Autodesk Inventor part; units mm, degrees
ref_plane "YZ Plane" through (0, 0, 0) normal (1, 0, 0) x (0, 1, 0)
ref_plane "XZ Plane" through (0, 0, 0) normal (0, 1, 0) x (-1, 0, 0)
ref_plane "XY Plane" through (0, 0, 0) normal (0, 0, 1) x (1, 0, 0)
sketch "Sketch1" plane through (0, 0, 0) normal (0, 0, 1) x (1, 0, 0)
  line L0 (-13.35, 6.2) -> (13.35, 6.2)
  line L1 (15.35, 4.2) -> (15.35, -4.2)
  line L2 (13.35, -6.2) -> (-13.35, -6.2)
  line L3 (-15.35, -4.2) -> (-15.35, 4.2)
  line L4 (-15.35, 6.2) -> (15.35, -6.2) construction
  line L5 (15.35, 6.2) -> (-15.35, -6.2) construction
  arc A0 (-13.35, 6.2) -> (-15.35, 4.2) centre (-13.35, 4.2) ccw
  arc A1 (15.35, 4.2) -> (13.35, 6.2) centre (13.35, 4.2) ccw
  arc A2 (13.35, -6.2) -> (15.35, -4.2) centre (13.35, -4.2) ccw
  arc A3 (-15.35, -4.2) -> (-13.35, -6.2) centre (-13.35, -4.2) ccw
  point P0 (0, 0)
  dimension "d0" = 12.4
  dimension "d1" = 30.7
  dimension "d2" = 2
extrude "Extrusion1" add sketch "Sketch1" along normal blind 1
sketch "Sketch2" plane through (0, 0, 1) normal (0, 0, 1) x (1, 0, 0)
  circle A0 centre (-12.495, 0) radius 1.55
  circle A1 centre (12.495, 0) radius 1.55
  line L0 (0, 0) -> (0, 2.0374)
  dimension "d5" = 3.1
  dimension "d6" = 24.99
extrude "Extrusion2" cut sketch "Sketch2" against normal through all
sketch "Sketch3" plane through (0, 0, 1) normal (0, 0, 1) x (1, 0, 0)
  line L0 (6.2132, 4.2657) -> (-6.2132, 4.2657)
  line L1 (-8.2003, 2.0385) -> (-7.7028, -2.3115)
  line L2 (-5.7157, -4.0843) -> (5.7157, -4.0843)
  line L3 (7.7028, -2.3115) -> (8.2003, 2.0385)
  line L4 (0, 0) -> (0, 9.8528)
  arc A0 (-6.2132, 4.2657) -> (-8.2003, 2.0385) centre (-6.2132, 2.2657) ccw
  arc A1 (8.2003, 2.0385) -> (6.2132, 4.2657) centre (6.2132, 2.2657) ccw
  arc A2 (5.7157, -4.0843) -> (7.7028, -2.3115) centre (5.7157, -2.0843) ccw
  arc A3 (-7.7028, -2.3115) -> (-5.7157, -4.0843) centre (-5.7157, -2.0843) ccw
  line L5 (6.2132, 2.2657) -> (-5.7157, -2.0843)
  line L6 (-6.2132, 2.2657) -> (5.7157, -2.0843)
  line L7 (-6.2132, 3.2657) -> (6.2132, 3.2657)
  arc A4 (7.2067, 2.1521) -> (6.2132, 3.2657) centre (6.2132, 2.2657) ccw
  line L8 (7.2067, 2.1521) -> (6.7092, -2.1979)
  arc A5 (5.7157, -3.0843) -> (6.7092, -2.1979) centre (5.7157, -2.0843) ccw
  line L9 (5.7157, -3.0843) -> (-5.7157, -3.0843)
  arc A6 (-6.7092, -2.1979) -> (-5.7157, -3.0843) centre (-5.7157, -2.0843) ccw
  line L10 (-6.7092, -2.1979) -> (-7.2067, 2.1521)
  arc A7 (-6.2132, 3.2657) -> (-7.2067, 2.1521) centre (-6.2132, 2.2657) ccw
  point P0 (8.455, 4.2657)
  point P1 (-8.455, 4.2657)
  point P2 (-7.5, -4.0843)
  point P3 (7.5, -4.0843)
  dimension "d9" = 8.35
  dimension "d10" = 16.91
  dimension "d11" = 15
  dimension "d12" = 2
  dimension "d15" = 1
extrude "Extrusion3" add sketch "Sketch3" along normal blind 6.1
properties part number "Dsub_9pin_female" material "Aluminum 6061"
Read the model definition and answer for the solid it produces. Units are mm, in the model's axes. A direction names the side the tool comes from. Coordinates: 2 decimals unless noted, no trailing zeros. Write each loop counter-clockwise with the first axis right and the second up, starting at its lowest first coordinate (ties: lowest second). Pieces come first, ordered by that corner, then holes. Notation, with made-up numbers: (42.25, 53.5) -> (82.25, 53.5) arc R32 cw to (82.25, 82.5) -> close; hole circle Ø8 at (33.5, 6.5). An arc over 180 degrees is marked (long way). Answer as a JSON object with one key per item and string values.
Q1. The part is cut by section D-D on x = -4. Give the vertices of the cut face in (y, z).
The answers:
{"outline": "(-6.2, 0) -> (6.2, 0) -> (6.2, 1) -> (4.27, 1) -> (4.27, 7.1) -> (3.27, 7.1) -> (3.27, 1) -> (-3.08, 1) -> (-3.08, 7.1) -> (-4.08, 7.1) -> (-4.08, 1) -> (-6.2, 1) -> close"}
Q2. The part is cut by section A-A on y = 1. Give the vertices of the cut face in (x, z).
The answers:
{"outline": "(-15.35, 0) -> (-13.68, 0) -> (-13.68, 1) -> (-15.35, 1) -> close; (-11.31, 0) -> (11.31, 0) -> (11.31, 1) -> (8.08, 1) -> (8.08, 7.1) -> (7.07, 7.1) -> (7.07, 1) -> (-7.07, 1) -> (-7.07, 7.1) -> (-8.08, 7.1) -> (-8.08, 1) -> (-11.31, 1) -> close; (13.68, 0) -> (15.35, 0) -> (15.35, 1) -> (13.68, 1) -> close"}
Q3. A tool of negligible diameter and unlimited length cuts with its end or side. For faces 4 (the cylindrical face through (-7.03, -3.59, 4.01)), 5 (the flat face through (0, 0, 1)), 6 (the cylindrical face through (-14.78, 5.6, 0.49)), from which of +Z, -Z, +X, -X, +Y, -Y can it reach the whole face along a straight path? Write none if from no direction.
The answers:
{"face 4": "+Z, -X, -Y", "face 5": "+Z", "face 6": "+Z, -Z, -X, +Y"}
Q4. The part is cut by section B-B on x = 11.5. Give the vertices of the cut face in (y, z), then the cut area to 3 significant figures.
The answers:
{"outline": "(-6.2, 0) -> (-1.19, 0) -> (-1.19, 1) -> (-6.2, 1) -> close; (1.19, 0) -> (6.2, 0) -> (6.2, 1) -> (1.19, 1) -> close", "area": "10.0 mm2"}
Q5. Consider line 1 (Y direction, x = 2, z = 6.25); line 2 (Z direction, x = 4, y = -4.25); line 3 (X direction, y = 1, z = 3). Determine where each line is inside the solid, lowest interval first. Write a range as [from, to].
The answers:
{"line 1": "y = [-4.08, -3.08], [3.27, 4.27]", "line 2": "z = [0, 1]", "line 3": "x = [-8.08, -7.07], [7.07, 8.08]"}
Q6. The part is cut by section C-C on z = 3.75. Give the vertices of the cut face in (x, y), then the cut area to 3 significant figures.
The answers:
{"outline": "(-8.2, 2.04) -> (-7.7, -2.31) arc R2 ccw to (-5.72, -4.08) -> (5.72, -4.08) arc R2 ccw to (7.7, -2.31) -> (8.2, 2.04) arc R2 ccw to (6.21, 4.27) -> (-6.21, 4.27) arc R2 ccw to start; hole (-7.21, 2.15) -> (-6.71, -2.2) arc R1 ccw to (-5.72, -3.08) -> (5.72, -3.08) arc R1 ccw to (6.71, -2.2) -> (7.21, 2.15) arc R1 ccw to (6.21, 3.27) -> (-6.21, 3.27) arc R1 ccw to start", "area": "42.0 mm2"}
Q7. Flat-ended cylindrical pins translate along their axes: pin 1 Ø2 at (x, z) = (1, 5.5) entering from +Y; pin 2 Ø1.8 at (x, z) = (1.5, 5) entering from -Y. Find the tip coordinate at first contact, or state that the pin passes through.
The answers:
{"pin 1": "stops at y = 4.27", "pin 2": "stops at y = -4.08"}
Q8. Determine the mould class of faces 1 (the flat face through (7.948, -0.167, 4.007)), 2 (the flat face through (1, 4, 7.1)), 3 (the flat face through (0, -3.084, 4)) for opening direction Y: pulls with the +Y half, pulls with the -Y half, needs draft (parallel to the pull), parting line crosses it, or undercut.
The answers:
{"face 1": "pulls with the -Y half", "face 2": "needs draft", "face 3": "undercut"}
